Here's how the part is built. I have some questions about the finished solid (model axes, mm). Face numbers are marked on the shaded views. A direction names the side the tool comes from. Give positions to 0.01 mm unless a question says otherwise; leave off trailing zeros. Loops run counter-clockwise (first coordinate to the right, second up) from the corner with the lowest first, then second, coordinate; pieces in that order, holes last.
Q1. Suppose I cut it at B-B (z = 33). List the corners of the cut face in (x, y) for me, and give its area (3 significant figures).
Q2. Thinking about a two-plate mould opening in X: for the marked faces 6, 7 and 8, which applies, pulls with the +X half, pulls with the -X half, needs draft (parallel to the pull), parting line crosses it, or undercut?
Q3. Suppose I cut it at A-A (x = 52). List the corners of the cut face in (y, z) for me, and give its area (3 significant figures).
Q4. For the marked faces 1, 2, 3, 4 and 5, which set-ups out of +Z, -Z, +X, -X, +Y, -Y let a thin tool reach every point of the face, with its end or its side?
Q5. I'm going to push flat-ended pins straight in: P1, Ø3, axis at y = 20.5, z = 96.5, coming from the +X side; P2, Ø8, axis at y = 28.75, z = 101.3, coming from the +X side; P3, Ø4, axis at y = 28.75, z = 85.3, coming from the +X side. Where does each tip first touch, or does it pass through?
Q6. Suppose I cut it at D-D (z = 101.3). List the corners of the cut face in (x, y) for me.
Q7. I need wall thicknesses on probe 1 along X at (y, z) = (49.5, 16.5); probe 2 along Z at (x, y) = (-7, 28); probe 3 along Z at (x, y) = (20.05, 28.75). Which ranges of each line are inside material? Lowest first, please.
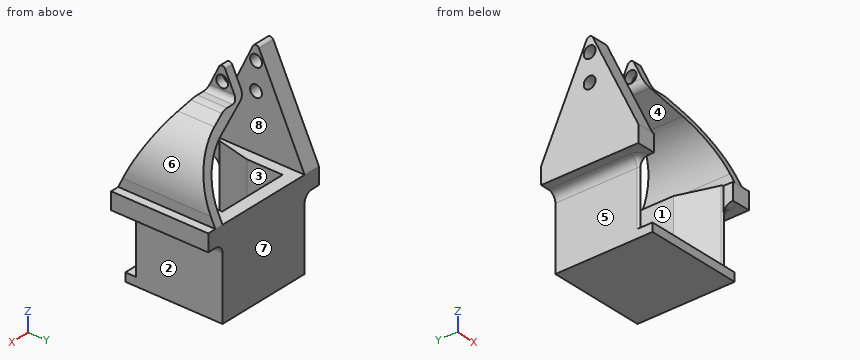
```python
from build123d import *

# Parameters (mm, degrees)
SKETCH2_W           = 57.5
SKETCH2_H           = 57.5
BOSS_EXTRUDE1_DEPTH = 5
SKETCH3_W           = 57.5
SKETCH3_H           = 57.5
SKETCH3_W_2         = 42.3
SKETCH3_H_2         = 42.3
BOSS_EXTRUDE2_DEPTH = 47.3
SKETCH4_W           = 70
SKETCH4_H           = 57.5
BOSS_EXTRUDE3_DEPTH = 10
SKETCH5_W           = 70
SKETCH5_H           = 57.5
BOSS_EXTRUDE4_DEPTH = 10
SKETCH6_W           = 35
SKETCH6_H           = 57.5
BOSS_EXTRUDE5_DEPTH = 38.75
SKETCH7_R           = 3.5
CUT_EXTRUDE1_DEPTH  = 144.086652068
SKETCH8_R           = 3.5
CUT_EXTRUDE2_DEPTH  = 144.086652068
FILLET1_R           = 30
CUT_EXTRUDE3_DEPTH  = 144.066205582
CUT_EXTRUDE4_REACH  = 109.048
CUT_EXTRUDE5_DEPTH  = 149.047084333
FILLET4_R           = 2
FILLET5_R           = 30
FILLET6_R           = 5
SKETCH12_W          = 11
SKETCH12_H          = 10
BOSS_EXTRUDE6_DEPTH = 10
FILLET7_R           = 1
FILLET8_R           = 5
CUT_EXTRUDE6_DEPTH  = 142.014244348
FILLET10_R          = 3
FILLET11_R          = 10


with BuildPart() as part:
    # Sketch2 → Boss-Extrude1 (new body)
    with BuildSketch(Plane.XY):
        with Locations((28.75, 28.75)):
            Rectangle(SKETCH2_W, SKETCH2_H)
    extrude(amount=BOSS_EXTRUDE1_DEPTH)

    # Sketch3 → Boss-Extrude2 (add)
    with BuildSketch(Plane.XY.offset(5)):
        with Locations((28.75, 28.75)):
            Rectangle(SKETCH3_W, SKETCH3_H)
        with Locations((27.525892101, 28.75)):
            Rectangle(SKETCH3_W_2, SKETCH3_H_2, mode=Mode.SUBTRACT)
    extrude(amount=BOSS_EXTRUDE2_DEPTH)

    # Sketch4 → Boss-Extrude3 (add)
    with BuildSketch(Plane.ZY):
        with Locations((77.3, 28.75)):
            Rectangle(SKETCH4_W, SKETCH4_H)
    extrude(amount=BOSS_EXTRUDE3_DEPTH)

    # Sketch5 → Boss-Extrude4 (add)
    with BuildSketch(Plane(origin=(57.5, 0, 0), x_dir=(0, 0, -1), z_dir=(1, 0, 0))):
        with Locations((-77.3, 28.75)):
            Rectangle(SKETCH5_W, SKETCH5_H)
    extrude(amount=BOSS_EXTRUDE4_DEPTH)

    # Sketch6 → Boss-Extrude5 (add)
    with BuildSketch(Plane.ZY.offset(-57.5)):
        with Locations((94.8, 28.75)):
            Rectangle(SKETCH6_W, SKETCH6_H)
    extrude(amount=BOSS_EXTRUDE5_DEPTH)

    # Sketch7 → Cut-Extrude1 (cut, through all)
    with BuildSketch(Plane(origin=(0, 0, 0), x_dir=(0, 0, -1), z_dir=(1, 0, 0))):
        with Locations((-101.3, 28.75)):
            Circle(SKETCH7_R)
        with Locations((-85.3, 28.75)):
            Circle(SKETCH7_R)
    extrude(amount=-CUT_EXTRUDE1_DEPTH, mode=Mode.SUBTRACT)

    # Sketch8 → Cut-Extrude2 (cut, through all)
    with BuildSketch(Plane(origin=(0, 0, 0), x_dir=(0, 0, -1), z_dir=(1, 0, 0))):
        with Locations((-101.3, 28.75)):
            Circle(SKETCH8_R)
    extrude(amount=CUT_EXTRUDE2_DEPTH, mode=Mode.SUBTRACT)

    # Fillet1
    # the kernel refuses this fillet: 30 mm, written as the material it takes off along each edge
    with BuildSketch(Plane(origin=(75, 57.5, 112.3), x_dir=(0, -1, 0), z_dir=(-1, 0, 0)), Plane(origin=(75, 0, 112.3), x_dir=(0, 0, -1), z_dir=(-1, 0, 0))) as fillet1_piece_1:
        with BuildLine():
            CenterArc((FILLET1_R, -FILLET1_R), FILLET1_R, 90, 90)
            Line((0, -FILLET1_R), (0, 0))
            Line((0, 0), (FILLET1_R, 0))
        make_face()
    extrude(amount=160, mode=Mode.SUBTRACT)
    with BuildSketch(Plane(origin=(142.5, 57.5, 112.3), x_dir=(0, -1, 0), z_dir=(-1, 0, 0)), Plane(origin=(142.5, 0, 112.3), x_dir=(0, 0, -1), z_dir=(-1, 0, 0))) as fillet1_piece_2:
        with BuildLine():
            CenterArc((FILLET1_R, -FILLET1_R), FILLET1_R, 90, 90)
            Line((0, -FILLET1_R), (0, 0))
            Line((0, 0), (FILLET1_R, 0))
        make_face()
    extrude(amount=198.75, mode=Mode.SUBTRACT)

    # Sketch9 → Cut-Extrude3 (cut, through all)
    with BuildSketch(Plane.XZ):
        Polygon((18.75, 77.3), (18.75, 94.8), (57.5, 77.3), align=None)
    extrude(amount=-CUT_EXTRUDE3_DEPTH, mode=Mode.SUBTRACT)

    # Cut-Extrude4: up to this face of the body (flat: up to its plane)
    cut_extrude4_end = Plane(part.part.faces().sort_by_distance((27.525892101, 28.75, 5))[0])
    # Sketch10 → Cut-Extrude4 (cut, up to the picked face)
    with BuildSketch(Plane.XY.offset(52.3), mode=Mode.PRIVATE) as cut_extrude4_sk1:
        Polygon((6.375892101, 28.75), (0, 0), (57.5, 0), (48.675892101, 28.75), align=None)
    cut_extrude4_tool1 = split(extrude(cut_extrude4_sk1.sketch, amount=-CUT_EXTRUDE4_REACH, mode=Mode.PRIVATE), bisect_by=cut_extrude4_end, keep=Keep.BOTH, mode=Mode.PRIVATE)
    add(cut_extrude4_tool1.solids().sort_by(Axis((28.169019, 13.645207, 52.3), (0, 0, -1)))[0], mode=Mode.SUBTRACT)

    # Sketch11 → Cut-Extrude5 (cut, through all)
    with BuildSketch(Plane(origin=(67.5, 0, 0), x_dir=(0, 0, -1), z_dir=(1, 0, 0))):
        with BuildLine():
            ThreePointArc((-82.3, 57.5), (-103.066559657, 49.150635095), (-112.273947021, 28.75))
            Line((-112.273947021, 28.75), (-52.3, 57.5))
            Line((-52.3, 57.5), (-82.3, 57.5))
        make_face()
        with BuildLine():
            Line((-52.3, 0), (-112.273947021, 28.75))
            ThreePointArc((-112.273947021, 28.75), (-103.066559657, 8.349364905), (-82.3, 0))
            Line((-82.3, 0), (-52.3, 0))
        make_face()
    extrude(amount=-CUT_EXTRUDE5_DEPTH, mode=Mode.SUBTRACT)

    # Fillet4
    fillet4_edges = [part.edges().sort_by_distance(p)[0] for p in [
        (-5, 28.75, 112.273947021),
        (43.125, 28.75, 112.273947021),
    ]]
    fillet(fillet4_edges, radius=FILLET4_R)

    # Fillet5
    fillet5_edges = [part.edges().sort_by_distance(p)[0] for p in [
        (57.5, 28.75, 77.3),
    ]]
    fillet(fillet5_edges, radius=FILLET5_R)

    # Fillet6
    # the kernel refuses this fillet: 5 mm, written as the material it takes off along each edge
    with BuildSketch(Plane(origin=(18.75, 12.302985171, 94.8), x_dir=(0.9113705996586746, 0, -0.4115867224264991), z_dir=(0, 1, 0))) as fillet6_piece_1:
        with BuildLine():
            CenterArc((FILLET6_R * 0.645635571077, -FILLET6_R), FILLET6_R, 90, 65.695450734)
            Line((-FILLET6_R * 0.265735028582, -FILLET6_R * 0.588413277574), (0, 0))
            Line((0, 0), (FILLET6_R * 0.645635571077, 0))
        make_face()
    extrude(amount=32.894029659, mode=Mode.SUBTRACT)

    # Sketch12 → Boss-Extrude6 (add)
    with BuildSketch(Plane.XZ):
        with Locations((-4.5, 47.3)):
            Rectangle(SKETCH12_W, SKETCH12_H)
        with Locations((62, 47.3)):
            Rectangle(SKETCH12_W, SKETCH12_H)
    extrude(amount=-BOSS_EXTRUDE6_DEPTH)

    # Fillet7
    # the kernel refuses this fillet: 1 mm, written as the material it takes off along each edge
    with BuildSketch(Plane(origin=(57.5, 0, 5), x_dir=(-0.29341611276772167, 0.9559848245491555, 0), z_dir=(0, 0, 1))) as fillet7_piece_1_section:
        with BuildLine():
            CenterArc((FILLET7_R * 6.66624885082, -FILLET7_R), FILLET7_R, 90, 162.937415162)
            Line((FILLET7_R * 6.37283273805, -FILLET7_R * 1.95598482455), (0, 0))
            Line((0, 0), (FILLET7_R * 6.66624885082, 0))
        make_face()
    fillet7_piece_1 = extrude(amount=53.965622127, mode=Mode.PRIVATE)
    fillet7_piece_1 = split(fillet7_piece_1, bisect_by=Plane(origin=(56.5, 4.962220999, 23.65), z_dir=(-1, 0, 0)), keep=Keep.TOP, mode=Mode.PRIVATE)
    add(fillet7_piece_1, mode=Mode.SUBTRACT)
    with BuildSketch(Plane(origin=(57.5, 0, 5), x_dir=(-0.29341611276772167, 0.9559848245491555, 0), z_dir=(0, 0, 1))) as fillet7_piece_2:
        with BuildLine():
            CenterArc((FILLET7_R * 6.66624885082, -FILLET7_R), FILLET7_R, 90, 162.937415162)
            Line((FILLET7_R * 6.37283273805, -FILLET7_R * 1.95598482455), (0, 0))
            Line((0, 0), (FILLET7_R * 6.66624885082, 0))
        make_face()
    extrude(amount=37.3, mode=Mode.SUBTRACT)
    with BuildSketch(Plane(origin=(0, 0, 65.119750157), x_dir=(0, 1, 0), z_dir=(0, 0, -1))) as fillet7_piece_3_section:
        with BuildLine():
            CenterArc((FILLET7_R * 9.12790006293, FILLET7_R), FILLET7_R, 102.504122974, 167.495877026)
            Line((FILLET7_R * 8.91139019581, FILLET7_R * 1.97628042971), (0, 0))
            Line((0, 0), (FILLET7_R * 9.12790006293, 0))
        make_face()
    fillet7_piece_3 = extrude(amount=60.119750157, mode=Mode.PRIVATE)
    fillet7_piece_3 = split(fillet7_piece_3, bisect_by=Plane(origin=(1, 7.031734734, 47.3), z_dir=(1, 0, 0)), keep=Keep.TOP, mode=Mode.PRIVATE)
    add(fillet7_piece_3, mode=Mode.SUBTRACT)
    with BuildSketch(Plane(origin=(0, 0, 42.3), x_dir=(0, 1, 0), z_dir=(0, 0, -1))) as fillet7_piece_4:
        with BuildLine():
            CenterArc((FILLET7_R * 9.12790006293, FILLET7_R), FILLET7_R, 102.504122974, 167.495877026)
            Line((FILLET7_R * 8.91139019581, FILLET7_R * 1.97628042971), (0, 0))
            Line((0, 0), (FILLET7_R * 9.12790006293, 0))
        make_face()
    extrude(amount=37.3, mode=Mode.SUBTRACT)

    # Fillet8
    fillet8_edges = [part.edges().sort_by_distance(p)[0] for p in [
        (0.292893219, 8.420793282, 42.3),
        (57.207106781, 5.95914207, 42.3),
        (0, 33.313950031, 42.3),
        (57.5, 32.083124425, 42.3),
    ]]
    fillet(fillet8_edges, radius=FILLET8_R)

    # Sketch13 → Cut-Extrude6 (cut, through all)
    with BuildSketch(Plane.XZ):
        with BuildLine():
            Line((32.827767642, 93.928540856), (23.75, 93.928540856))
            Line((23.75, 93.928540856), (23.75, 98.028177855))
            Line((23.75, 98.028177855), (23.75, 108.511784994))
            Line((23.75, 108.511784994), (23.75, 111.823529661))
            Line((23.75, 111.823529661), (71.506891102, 111.823529661))
            Line((71.506891102, 111.823529661), (71.506891102, 52.3))
            Line((71.506891102, 52.3), (62.5, 52.3))
            Line((62.5, 52.3), (62.5, 57.930932868))
            ThreePointArc((62.5, 57.930932868), (56.904028083, 76.915219331), (41.905535285, 89.828903856))
            Line((41.905535285, 89.828903856), (32.827767642, 93.928540856))
        make_face()
    extrude(amount=-CUT_EXTRUDE6_DEPTH, mode=Mode.SUBTRACT)

    # Fillet10
    fillet10_edges = [part.edges().sort_by_distance(p)[0] for p in [
        (23.75, 28.75, 93.928540856),
    ]]
    fillet(fillet10_edges, radius=FILLET10_R)

    # Fillet11
    fillet11_edges = [part.edges().sort_by_distance(p)[0] for p in [
        (32.827767642, 28.75, 93.928540856),
    ]]
    fillet(fillet11_edges, radius=FILLET11_R)


solid = part.part
```
Solutions:
1. outline: (0, 9.13) arc R1 ccw to (1.98, 8.91) - (6.38, 28.75) - (6.38, 49.9) - (48.68, 49.9) - (48.68, 28.75) - (55.54, 6.37) arc R1 ccw to (57.5, 6.67) - (57.5, 57.5) - (0, 57.5) - close
1. area: 964 mm2
2. face 6: pulls with the +X half
2. face 7: needs draft
2. face 8: undercut
3. outline: (0, 0) - (57.5, 0) - (57.5, 52.3) - (17.92, 52.3) - (17.92, 5) - (0, 5) - close; (11, 75.24) - (46.5, 75.24) - (42.82, 82.93) - (14.68, 82.93) - close
3. area: 2,400 mm2
4. face 1: -Y
4. face 2: -Z, +X, +Y, -Y
4. face 3: +Z, -Y
4. face 4: +Y, -Y
4. face 5: -Z, -X, +Y, -Y
5. P1: stops at x = 24.45
5. P2: stops at x = 23.75
5. P3: stops at x = 51.61
6. outline: (-10, 23.49) - (0, 23.49) - (0, 25.25) - (-10, 25.25) - close; (-10, 32.25) - (0, 32.25) - (0, 34.01) - (-10, 34.01) - close; (18.75, 23.49) - (23.75, 23.49) - (23.75, 25.25) - (18.75, 25.25) - close; (18.75, 32.25) - (23.75, 32.25) - (23.75, 34.01) - (18.75, 34.01) - close
7. probe 1: x = 0 to 6.38, 48.68 to 57.5
7. probe 2: z = 42.3 to 81.88, 88.72 to 97.88, 104.72 to 109.5
7. probe 3: z = 0 to 5, 94.67 to 97.8, 104.8 to 109.65
